Read the model definition and answer for the solid it produces. Units are mm, in the model's axes. Coordinates: 2 decimals unless noted, no trailing zeros. Order: outer loops, then holes, each group sorted by start corner. A loop starts at its lowest first (then second) coordinate and runs counter-clockwise, first axis right, second up. Notation, with made-up numbers: (7, 23.25) - (45, 23.25) arc R22 cw to (45, 57.25) - close; hole circle Ø1 at (-24, -27.5). An arc over 180 degrees is marked (long way). Use one line per item in the form item = value.
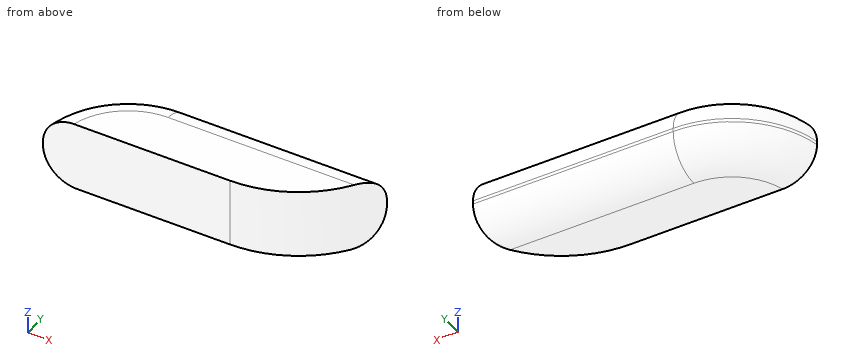
```python
from build123d import *

# Parameters (mm, degrees)
F1_DEPTH = 50.8
F2_R     = 22.86
F3_R     = 25.4


with BuildPart() as f1:
    # F0 (on Top) → F1 (new body)
    with BuildSketch(Plane.XY):
        with BuildLine():
            ThreePointArc((13.428768, 121.414845), (-33.346659, 104.181794), (-57.761153, 60.720879))
            Line((-57.761153, 60.720879), (83.249649, 60.720879))
            ThreePointArc((83.249649, 60.720879), (133.949731, 77.570215), (164.479175, 121.414845))
            Line((164.479175, 121.414845), (13.428768, 121.414845))
        make_face()
    extrude(amount=F1_DEPTH)

    # F2
    f2_edges = [f1.edges().sort_by_distance(p)[0] for p in [
        (-33.346659, 104.181794, 50.8),
        (88.953971, 121.414845, 50.8),
    ]]
    fillet(f2_edges, radius=F2_R)

    # F3
    f3_edges = [f1.edges().sort_by_distance(p)[0] for p in [
        (88.953971, 121.414845, 0),
        (-33.346659, 104.181794, 0),
    ]]
    fillet(f3_edges, radius=F3_R)


solid = f1.part
```
(1) Section B-B, the plane z = 46.5 is taken. Write down the section's boundary in (x, y), then the cut area to 3 significant figures.
Answer list:
outline = (-48.11, 60.72) - (83.25, 60.72) arc R84.7 ccw to (161.04, 111.9) - (13.43, 111.9) arc R62.58 ccw to start
area = 8,810 mm2
(2) Section C-C, the plane x = 110 is taken. Write down the section's boundary in (y, z), then the cut area to 3 significant figures.
Answer list:
outline = (65.06, 0) - (96.01, 0) arc R25.4 ccw to (121.41, 25.4) - (121.41, 27.94) arc R22.86 ccw to (98.55, 50.8) - (65.06, 50.8) - close
area = 2,610 mm2
(3) Given pin 1 Ø12 at (x, y) = (77.5, 106.5) entering from +Z; pin 2 Ø6 at (y, z) = (89, 17) entering from -X; pin 3 Ø4 at (y, z) = (102.5, 41) entering from -X, each flat-ended and moving along its own axis, determine where each tip first touches the part or whether it passes through.
Answer list:
pin_1 = 50.72
pin_2 = -47.28
pin_3 = -32.07
(4) Section D-D, the plane z = 18 is taken. Write down the section's boundary in (x, y).
Answer list:
outline = (-56.65, 60.72) - (83.25, 60.72) arc R84.7 ccw to (164.15, 120.31) - (13.43, 120.31) arc R71 ccw to start
(5) Section A-A, the plane x = 77 is taken. Write down the section's boundary in (y, z).
Answer list:
outline = (60.72, 0) - (96.01, 0) arc R25.4 ccw to (121.41, 25.4) - (121.41, 27.94) arc R22.86 ccw to (98.55, 50.8) - (60.72, 50.8) - close
(6) Straight lines are drawn through the part: L1, parallel to Z at x = 84, y = 97.5; L2, parallel to Z at x = 134.5, y = 114; L3, parallel to Y at x = 141.5, z = 38. For each, find the intervals that lie inside material, in ascending order.
Answer list:
L1 = 0.04 to 50.8
L2 = 7.46 to 44.79
L3 = 83.93 to 119.08
